Check sheet for the modelled part. Datum: model origin and axes. Units: mm. A direction names the side the tool comes from. Round coordinates to 2 decimals unless told otherwise and drop trailing zeros. Write each loop counter-clockwise with the first axis right and the second up, starting at its lowest first coordinate (ties: lowest second). Pieces come first, ordered by that corner, then holes. Notation, with made-up numbers: M 44.5,48.25 L 87.5,48.25 A21 ccw 87.5,72.25 Z; hole C 28,32 d10. An arc over 180 degrees is marked long. One line per item, written item: value.
from build123d import *

# Parameters (mm, degrees)
CUT_EXTRUDE1_DEPTH           = 21
CUT_EXTRUDE1_DEPTH_BACK      = 21
CUT_EXTRUDE2_DEPTH           = 21
CUT_EXTRUDE2_DEPTH_BACK      = 21
CUT_EXTRUDE3_DEPTH           = 21
CUT_EXTRUDE3_DEPTH_BACK      = 21
SKETCH5_W                    = 26
SKETCH5_H                    = 5
CUT_REVOLVE3_ANGLE           = 90
CUT_REVOLVE3_OTHER_WAY_ANGLE = 90


with BuildPart() as part:
    # Sketch1 → Revolve1 (revolve)
    with BuildSketch(Plane(origin=(0, 0, 0), x_dir=(0, 0, -1), z_dir=(1, 0, 0))):
        with BuildLine():
            Line((-12, 0), (-12, 20))
            Line((-12, 20), (22.387495374, 20))
            Line((22.387495374, 20), (25, 10.25))
            ThreePointArc((25, 10.25), (25.366116524, 9.366116524), (26.25, 9))
            Line((26.25, 9), (39.1, 9))
            ThreePointArc((39.1, 9), (39.736396103, 8.736396103), (40, 8.1))
            Line((40, 8.1), (40, 0))
            Line((40, 0), (-12, 0))
        make_face()
    revolve(axis=Axis((0, 0, -40), (0, 0, 1)))

    # Sketch2 → Cut-Extrude1 (cut, two sides)
    with BuildSketch(Plane(origin=(0, 0, 0), x_dir=(1, 0, 0), z_dir=(0, 1, 0))) as cut_extrude1_sk:
        Polygon((-5, 19), (-5, -13), (5, -13), (5, 19), (4, 20), (-4, 20), align=None)
    extrude(amount=CUT_EXTRUDE1_DEPTH, mode=Mode.SUBTRACT)
    extrude(cut_extrude1_sk.sketch, amount=-CUT_EXTRUDE1_DEPTH_BACK, mode=Mode.SUBTRACT)

    # Sketch3 → Cut-Extrude2 (cut, two sides)
    with BuildSketch(Plane(origin=(0, 0, 0), x_dir=(0, 0, -1), z_dir=(1, 0, 0))) as cut_extrude2_sk:
        Polygon((-33, -30), (40, -30), (40, -10), (-13, -10), (-13, 10), (40, 10), (40, 30), (-33, 30), align=None)
    extrude(amount=CUT_EXTRUDE2_DEPTH, mode=Mode.SUBTRACT)
    extrude(cut_extrude2_sk.sketch, amount=-CUT_EXTRUDE2_DEPTH_BACK, mode=Mode.SUBTRACT)

    # Sketch4 → Cut-Extrude3 (cut, two sides)
    with BuildSketch(Plane(origin=(0, 0, 0), x_dir=(1, 0, 0), z_dir=(0, 1, 0))) as cut_extrude3_sk:
        Polygon((-30, -33), (30, -33), (30, 40), (10, 40), (10, -13), (-10, -13), (-10, 40), (-30, 40), align=None)
    extrude(amount=CUT_EXTRUDE3_DEPTH, mode=Mode.SUBTRACT)
    extrude(cut_extrude3_sk.sketch, amount=-CUT_EXTRUDE3_DEPTH_BACK, mode=Mode.SUBTRACT)

    # Sketch5 → Cut-Revolve1 (revolve, cut)
    with BuildSketch(Plane.XY):
        with Locations((0, 2.5)):
            Rectangle(SKETCH5_W, SKETCH5_H)
    revolve(axis=Axis((13, 0, 0), (-1, 0, 0)), mode=Mode.SUBTRACT)

    # Sketch6 → Cut-Revolve2 (revolve, cut)
    with BuildSketch(Plane(origin=(0, 0, 0), x_dir=(0, 0, -1), z_dir=(1, 0, 0))):
        Polygon((18.9, 0), (18.9, 4.3235), (39.4235, 4.3235), (40.1, 5), (40.1, 0), align=None)
    revolve(axis=Axis((0, 0, -40.1), (0, 0, 1)), mode=Mode.SUBTRACT)

    # Sketch7 → Cut-Revolve3 (revolve, cut)
    with BuildSketch(Plane(origin=(0, 0, 0), x_dir=(1, 0, 0), z_dir=(0, 1, 0))):
        Polygon((-12, -8.000813089), (-12, -31.094823856), (0, -38.023027087), (12, -31.094823856), (12, -8.000813089), (0, -14.929016319), align=None)
    revolve(axis=Axis((-12, 0, -20), (1, 0, 0)), revolution_arc=CUT_REVOLVE3_ANGLE, mode=Mode.SUBTRACT)

    # Sketch7 → Cut-Revolve3 other way (revolve, cut)
    with BuildSketch(Plane(origin=(0, 0, 0), x_dir=(1, 0, 0), z_dir=(0, 1, 0))):
        Polygon((-12, -8.000813089), (-12, -31.094823856), (0, -38.023027087), (12, -31.094823856), (12, -8.000813089), (0, -14.929016319), align=None)
    revolve(axis=Axis((-12, 0, -20), (-1, 0, 0)), revolution_arc=CUT_REVOLVE3_OTHER_WAY_ANGLE, mode=Mode.SUBTRACT)


solid = part.part
Q1. Sectioned sample at C-C on z = -12.5. Enter the section's corners in (x, y), and give its area (3 significant figures).
Completed:
outline: M -10,-10 L -5,-10 L -5,10 L -10,10 Z; M 5,-10 L 10,-10 L 10,10 L 5,10 Z
area: 200 mm^2
Q2. Sectioned sample at B-B on y = 0. State how many separate pieces and enclosed holes the cut face has, and give its area (3 significant figures).
Completed:
separate pieces: 4
enclosed holes: 0
area: 404 mm^2
Q3. Sectioned sample at D-D on x = 0. Enter the section's corners in (y, z).
Completed:
outline: M -10,-25.03 A1.25 cw -9,-26.25 L -9,-39.1 A0.9 ccw -8.1,-40 L -4.9,-40 L -4.32,-39.42 L -4.32,-20 L -10,-20 Z; M 4.32,-39.42 L 4.9,-40 L 8.1,-40 A0.9 ccw 9,-39.1 L 9,-26.25 A1.25 cw 10,-25.03 L 10,-20 L 4.32,-20 Z
Q4. Sectioned sample at A-A on z = 0. Enter the section's corners in (x, y), and give its area (3 significant figures).
Completed:
outline: M -10,-10 L -5,-10 L -5,-5 L -10,-5 Z; M -10,5 L -5,5 L -5,10 L -10,10 Z; M 5,-10 L 10,-10 L 10,-5 L 5,-5 Z; M 5,5 L 10,5 L 10,10 L 5,10 Z
area: 100 mm^2
Q5. Depth check by flat-ended pin: P1, Ø1, axis at x = 2, y = -2, coming from the +Z side; P2, Ø2.5, axis at x = -1.5, y = 4, coming from the +Z side; P3, Ø3, axis at y = 2.5, z = -30.5, coming from the -X side. Enter the tip coordinate at first touch or a pass-through.
Completed:
P1: through
P2: z = -20
P3: x = -8.94
Q6. Draft check along Y on faces 4 (the flat face through (-10, 0, -8)), 5 (the cylindrical face through (2.63, -3.43, -29.66)), 6 (the cylindrical face through (-7.46, -1.08, 4.88)), 7 (the conical face through (-7.93, 8.056, -24.718)). Enter one of: pulls with the +Y half, pulls with the -Y half, needs draft (parallel to the pull), parting line crosses it, or undercut.
Completed:
face 4: needs draft
face 5: undercut
face 6: undercut
face 7: pulls with the +Y half
Q7. Scan lines: line 1 (X direction, y = 0, z = -33); line 2 (X direction, y = 9, z = -14). Record each from-to range of solid material in increasing order. Write a range as [from, to].
Completed:
line 1: [-9, -4.32], [4.32, 9]
line 2: [-10, -5], [5, 10]
Q8. Access from +Z, -Z, +X, -X, +Y, -Y to the whole of each face (thin tool, end or side, straight path). Record for faces 1 (the conical face through (7.5, 0.2, 10.6)), 2 (the cylindrical face through (-8.923, -1.172, -32.765)), 3 (the flat face through (5, 0, -7)).
Completed:
face 1: +Z, +X
face 2: -Z
face 3: +Z, +Y, -Y
